Input: dimensioned drawing with shaded views. Units: mm. Origin: part minimum x, y, z. A direction names the side the tool comes from. Give positions to 0.01 mm unless a question says otherwise; leave off trailing zeros. Order: outer loops, then holes, each group sorted by start corner. A loop starts at its lowest first (then second) coordinate and runs counter-clockwise, first axis right, second up. Notation, with made-up numbers: (23, -21.5) - (47, -21.5) arc R26 ccw to (47, 0.5) - close; hole circle Ø2 at (41.5, 57.25). An arc over 180 degrees is marked (long way). Answer as CSV lines item,"result".
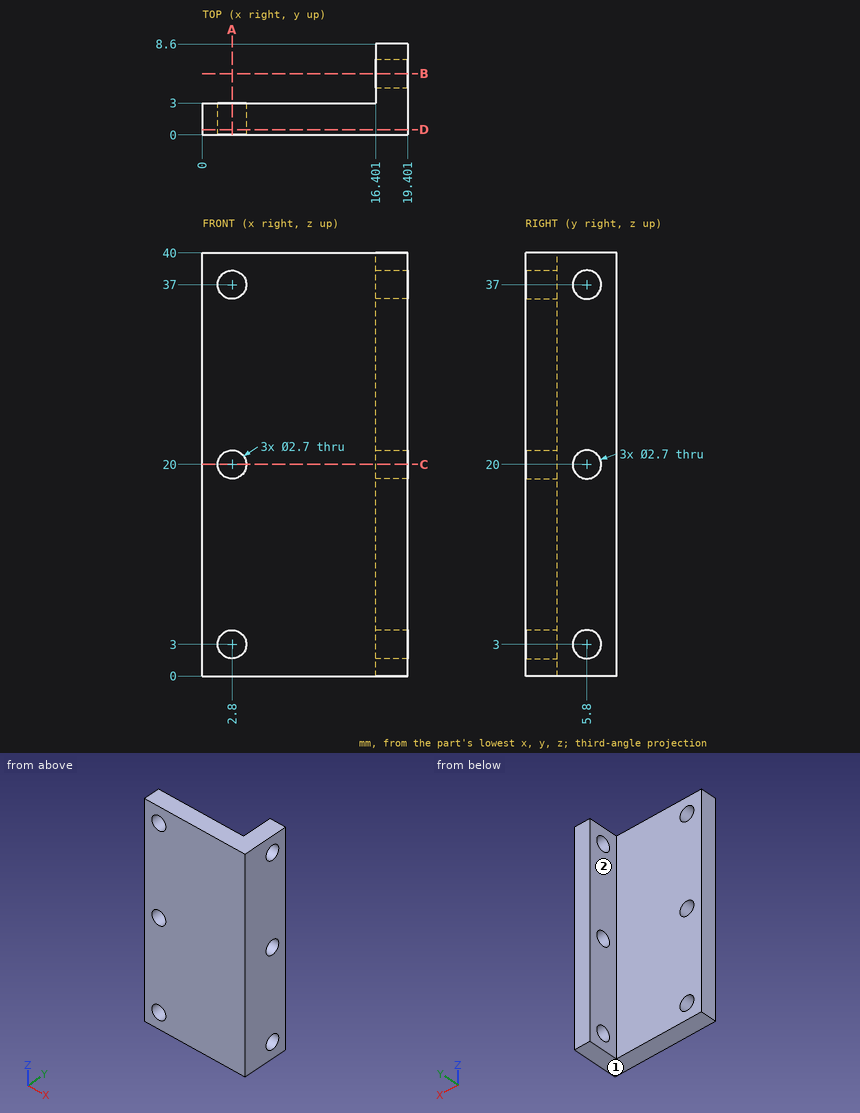
(1) Cut plane A-A (x = 2.8). Return loops of the section in (y, z), then the cut area to 3 significant figures.
Completed:
outline,"(0, 0) - (3, 0) - (3, 1.65) - (0, 1.65) - close; (0, 4.35) - (3, 4.35) - (3, 18.65) - (0, 18.65) - close; (0, 21.35) - (3, 21.35) - (3, 35.65) - (0, 35.65) - close; (0, 38.35) - (3, 38.35) - (3, 40) - (0, 40) - close"
area,"95.7 mm²"
(2) Cut plane B-B (y = 5.8). Return loops of the section in (x, z).
Completed:
outline,"(16.4, 0) - (19.4, 0) - (19.4, 1.65) - (16.4, 1.65) - close; (16.4, 4.35) - (19.4, 4.35) - (19.4, 18.65) - (16.4, 18.65) - close; (16.4, 21.35) - (19.4, 21.35) - (19.4, 35.65) - (16.4, 35.65) - close; (16.4, 38.35) - (19.4, 38.35) - (19.4, 40) - (16.4, 40) - close"
(3) Contact query for flat-ended pins moving along their axis: pin 1 (4.5 mm diameter, centred on x = 2.8, z = 37, fed in from -Y); pin 2 (1.5 mm diameter, centred on x = 6.5, z = 34, fed in from +Y); pin 3 (3 mm diameter, centred on y = 5.8, z = 37, fed in from -X). Output: stop coordinate, or through.
Completed:
pin 1,"y = 0"
pin 2,"y = 3"
pin 3,"x = 16.4"
(4) Access query for the marked faces 1 and 2. Directions: +Z, -Z, +X, -X, +Y, -Y. A direction counts if a zero-diameter tool reaches every point of the face in a straight line with its end or side. Return the directions, or none.
Completed:
face 1,"-Z, +X, -X, +Y, -Y"
face 2,"+Z, -Z, -X, +Y"
(5) Ray query, line 1 (Z direction, x = 2.8, y = 2.1); line 2 (Y direction, x = 3.75, z = 7); line 3 (X direction, y = 1.25, z = 37). Return the intervals inside material, ascending. Write a range as from..to.
Completed:
line 1,"0..1.65, 4.35..18.65, 21.35..35.65, 38.35..40"
line 2,"0..3"
line 3,"0..1.45, 4.15..19.4"
(6) Cut plane D-D (y = 0.5). Return loops of the section in (x, z).
Completed:
outline,"(0, 0) - (19.4, 0) - (19.4, 40) - (0, 40) - close; hole circle Ø2.7 at (2.8, 3); hole circle Ø2.7 at (2.8, 20); hole circle Ø2.7 at (2.8, 37)"
(7) Cut plane C-C (z = 20). Return loops of the section in (x, y), then the cut area to 3 significant figures.
Completed:
outline,"(0, 0) - (1.45, 0) - (1.45, 3) - (0, 3) - close; (4.15, 0) - (19.4, 0) - (19.4, 4.45) - (16.4, 4.45) - (16.4, 3) - (4.15, 3) - close; (16.4, 7.15) - (19.4, 7.15) - (19.4, 8.6) - (16.4, 8.6) - close"
area,"58.8 mm²"
